```python
from build123d import *

# Parameters (mm, degrees)
SKETCH1_R           = 3.96875
BOSS_EXTRUDE1_DEPTH = 50.8
SKETCH6_R           = 4.7625
CUT_EXTRUDE3_DEPTH  = 12.7
FILLET2_R           = 12.7


with BuildPart() as part:
    # Sketch1 → Boss-Extrude1 (new body)
    with BuildSketch(Plane.XY):
        with BuildLine():
            ThreePointArc((7.14375, 0), (0, 7.14375), (-7.14375, 0))
            Line((-7.14375, 0), (-7.14375, -7.14375))
            Line((-7.14375, -7.14375), (111.91875, -7.14375))
            Line((111.91875, -7.14375), (111.91875, -3.96875))
            Line((111.91875, -3.96875), (7.14375, -3.96875))
            Line((7.14375, -3.96875), (7.14375, 0))
        make_face()
        Circle(SKETCH1_R, mode=Mode.SUBTRACT)
    extrude(amount=BOSS_EXTRUDE1_DEPTH)

    # Sketch6 → Cut-Extrude3 (cut)
    with BuildSketch(Plane(origin=(0, -3.96875, 0), x_dir=(1, 0, 0), z_dir=(0, 1, 0))):
        with Locations((19.84375, -25.4)):
            Circle(SKETCH6_R)
        with Locations((99.21875, -25.4)):
            Circle(SKETCH6_R)
    extrude(amount=-CUT_EXTRUDE3_DEPTH, mode=Mode.SUBTRACT)

    # Fillet2
    fillet2_edges = [part.edges().sort_by_distance(p)[0] for p in [
        (111.91875, -5.55625, 0),
        (111.91875, -5.55625, 50.8),
    ]]
    fillet(fillet2_edges, radius=FILLET2_R)


solid = part.part
```
Check sheet for the modelled part. Datum: model origin and axes. Units: mm. A direction names the side the tool comes from. Round coordinates to 2 decimals unless told otherwise and drop trailing zeros. Order: outer loops, then holes, each group sorted by start corner. A loop starts at its lowest first (then second) coordinate and runs counter-clockwise, first axis right, second up.
1) Mould release check, pull along X, two halves, no side actions. Record for faces 3 (the cylindrical face through (0.16, 7.14, 25.04)), 4 (the cylindrical face through (-0.86, -3.874, 25.044)), 5 (the cylindrical face through (108.1, -5.53, 47.18)): +X half, -X half, draft (parallel to the pull), parting line (faces both ways), or undercut.
2) Section check A-A (x = 0). Record the boundary of the cut face in (y, z), and give its area (3 significant figures).
3) Section check C-C (y = -5.75). Record the boundary of the cut face in (x, z) (1 decimal).
4) Section check D-D (z = 18.5). Record the boundary of the cut face in (x, y), and give its area (3 significant figures).
5) Scan lines: line 1 (X direction, y = -6.4, z = 25.4); line 2 (Y direction, x = 0, z = 40); line 3 (Y direction, x = 94.5, z = 3.5). Record each from-to range of solid material in increasing order.
6) Section check B-B (z = 25.4). Record the boundary of the cut face in (x, y), and give its area (3 significant figures).
7) Go/stop test with flat-tipped pins: pin 1 Ø5 at (x, y) = (0, 0) entering from +Z; pin 2 Ø3 at (y, z) = (1.5, 45) entering from +X. Record where each tip stops, or that it passes through.
8) Tool access check on faces 1 (the flat face through (111.919, -6, 25)), 2 (the flat face through (60, -3.969, 25)). Record the directions out of +Z, -Z, +X, -X, +Y, -Y that give a thin tool (end or side, any length) a straight path to the whole face; none if there is none.
Result:
1. face 3: parting line
1. face 4: undercut
1. face 5: +X half
2. outline: (-7.14, 0) - (-3.97, 0) - (-3.97, 50.8) - (-7.14, 50.8) - close; (3.97, 0) - (7.14, 0) - (7.14, 50.8) - (3.97, 50.8) - close
2. area: 323 mm2
3. outline: (-7.1, 0) - (99.2, 0) arc R12.7 ccw to (111.9, 12.7) - (111.9, 38.1) arc R12.7 ccw to (99.2, 50.8) - (-7.1, 50.8) - close; hole circle Ø9.5 at (19.8, 25.4); hole circle Ø9.5 at (99.2, 25.4)
4. outline: (-7.14, -7.14) - (111.92, -7.14) - (111.92, -3.97) - (7.14, -3.97) - (7.14, 0) arc R7.14 ccw to (-7.14, 0) - close; hole circle Ø7.94 at (0, 0)
4. area: 465 mm2
5. line 1: x = -7.14 to 15.08, 24.61 to 94.46, 103.98 to 111.92
5. line 2: y = -7.14 to -3.97, 3.97 to 7.14
5. line 3: y = -7.14 to -3.97
6. outline: (-7.14, -7.14) - (15.08, -7.14) - (15.08, -3.97) - (7.14, -3.97) - (7.14, 0) arc R7.14 ccw to (-7.14, 0) - close; (24.61, -7.14) - (94.46, -7.14) - (94.46, -3.97) - (24.61, -3.97) - close; (103.98, -7.14) - (111.92, -7.14) - (111.92, -3.97) - (103.98, -3.97) - close; hole circle Ø7.94 at (0, 0)
6. area: 405 mm2
7. pin 1: passes through
7. pin 2: stops at x = 7.14
8. face 1: +Z, -Z, +X, +Y, -Y
8. face 2: +Z, -Z, +X, +Y
